Work out the finished part from the listing and answer in its coordinate system (mm). A direction names the side the tool comes from. Give positions to 0.01 mm unless a question says otherwise; leave off trailing zeros. Loops run counter-clockwise (first coordinate to the right, second up) from the corner with the lowest first, then second, coordinate; pieces in that order, holes last.
Autodesk Inventor part; units mm, degrees
ref_plane "YZ Plane" through (0, 0, 0) normal (1, 0, 0) x (0, 1, 0)
ref_plane "XZ Plane" through (0, 0, 0) normal (0, 1, 0) x (-1, 0, 0)
ref_plane "XY Plane" through (0, 0, 0) normal (0, 0, 1) x (1, 0, 0)
sketch "Skizze1" plane through (0, 0, 0) normal (0, 0, 1) x (1, 0, 0)
  line L0 (3.6, 12) -> (48, 12)
  line L1 (48, 12) -> (48, -12)
  line L2 (48, -12) -> (3.6, -12)
  line L3 (-189.6, 0) -> (87.6, 0)
  line L4 (-1, 15) -> (-10, 28.5)
  line L5 (-1, -15) -> (-10, -28.5)
  line L6 (-10, -28.5) -> (-14, -28.5)
  line L7 (-10, 28.5) -> (-14, 28.5)
  arc A0 (-11.6616, 21.5053) -> (-14, 28.5) centre (-33.4005, 18.1259) ccw
  arc A1 (-14, -28.5) -> (-11.6616, -21.5053) centre (-33.4005, -18.1259) ccw
  arc A2 (-11.6616, -21.5053) -> (-11.6616, 21.5053) centre (-150, 0) ccw
  line L8 (-10, 28.5) -> (-10, -28.5) construction
  line L9 (0, 40.0382) -> (0, -40.0382)
  line L10 (-2, 12.5) -> (-2, -9.8115) construction
  arc A3 (0, 12) -> (3.6, 12) centre (1.8, 12) ccw
  arc A4 (3.6, -12) -> (0, -12) centre (1.8, -12) ccw
  line L11 (0, 12) -> (0, 15)
  line L12 (0, 15) -> (-1, 15)
  line L13 (0, -12) -> (0, -15)
  line L14 (0, -15) -> (-1, -15)
  point P0 (0, 0)
  dimension "d2" = 24
  dimension "d51" = 22
  dimension "d52" = 140
  dimension "d54" = 4
  dimension "d55" = 57
  dimension "d59" = 8
  dimension "d60" = 2
  dimension "d64" = 0
  dimension "d73" = 1.8
  dimension "d75" = 48
  dimension "d76" = 30
  dimension "d77" = 1
extrude "Extrusion1" add sketch "Skizze1" along normal blind 12
sketch "Skizze8" plane through (0, 0, 12) normal (0, 0, 1) x (1, 0, 0)
  line L0 (-189.6, 0) -> (87.6, 0)
  arc A0 (-11.6616, -21.5053) -> (-11.6616, 21.5053) centre (-150, 0) ccw
  line L1 (-1, 15) -> (-10, 28.5)
  line L2 (-11.2277, 18.5) -> (-3.3333, 18.5) construction
  point P0 (0, 0)
  point P1 (-5.7805, 18.5)
  point P2 (-5.7805, -18.5)
  point P3 (-7.2805, 18.5)
  dimension "d65" = 18.5
  dimension "d80" = 1.5
hole "Bohrung4" at (-5.7805, 18.5, 12) at (-5.7805, -18.5, 12) direction (0, 0, -1) diameter 1.567 end through all counterbore diameter 5.5 counterbore depth 7
sketch "Skizze2" plane through (0, 0, 0) normal (0, 0, -1) x (-1, 0, 0)
  line L0 (-48, -12) -> (-3.6, -12)
  line L1 (-48, 12) -> (-48, -12)
  line L2 (-48, 12) -> (-3.6, 12)
  line L3 (0, -12) -> (-48, -12)
  line L4 (-48, -12) -> (-48, 12)
  line L5 (-48, 12) -> (0, 12)
  line L6 (-3.6, 12) -> (-48, 12)
  line L7 (0, 12) -> (0, -12)
  point P0 (0, 0)
  point P1 (0, -12.5)
  point P2 (0, 12.5)
  point P3 (-3.6, -12)
extrude "Extrusion2" cut sketch "Skizze2" against normal blind 8
sketch "Skizze3" plane through (0, 0, 8) normal (0, 0, -1) x (-1, 0, 0)
  line L0 (-3.6, -12) -> (-48, -12)
  line L1 (-48, -12) -> (-48, 12)
  line L2 (-48, 12) -> (-3.6, 12)
  line L3 (-48, -12) -> (-44, -12)
  line L4 (-44, -12) -> (-44, 12)
  line L5 (-44, 12) -> (-48, 12)
  line L6 (-48, 12) -> (-48, -12)
  point P0 (0, 0)
  point P1 (0, -12.5)
  point P2 (0, 12.5)
  point P3 (10, -12.5)
  point P4 (-3.6, 12)
  dimension "d9" = 4
extrude "Extrusion3" cut sketch "Skizze3" against normal blind 2
sketch "Skizze4" plane through (0, 0, 12) normal (0, 0, 1) x (1, 0, 0)
  line L0 (48, -12) -> (48, 12)
  line L1 (-26.4, 0) -> (60.4, 0)
  point P0 (0, 0)
  point P1 (46, 0)
  dimension "d12" = 2
hole "Bohrung1" at (46, 0, 12) direction (0, 0, -1) diameter 2 end through all
pattern_linear "Rechteckige Anordnung1" count 5 spacing 5 along (0, 1, 0) of "Bohrung1" first direction both ways yes
sketch "Skizze7" plane through (0, 0, 12) normal (0, 0, 1) x (1, 0, 0)
  line L0 (-1, 15) -> (-3.061, 18.0915)
  line L1 (-10, 28.5) -> (-14, 28.5)
  arc A0 (-11.6616, 21.5053) -> (-14, 28.5) centre (-33.4005, 18.1259) ccw
  arc A1 (-11.6616, -21.5053) -> (-11.6616, 21.5053) centre (-150, 0) ccw
  arc A2 (-14, -28.5) -> (-11.6616, -21.5053) centre (-33.4005, -18.1259) ccw
  line L2 (-14, -28.5) -> (-10, -28.5)
  line L3 (-10, -28.5) -> (-5.1116, -21.1674)
  line L4 (3.6, -12) -> (48, -12)
  line L5 (48, -12) -> (48, 12)
  line L6 (48, 12) -> (3.6, 12)
  line L7 (-3, 28.5) -> (-14, 28.5)
  line L8 (-14, 28.5) -> (-14, -28.5)
  line L9 (-14, -28.5) -> (-3, -28.5)
  line L10 (-3, -28.5) -> (-3, 28.5)
  line L11 (-10, 28.5) -> (-14, 28.5)
  line L12 (-14, -28.5) -> (-10, -28.5)
  line L13 (0, 12) -> (0, 15)
  line L14 (0, 15) -> (-1, 15)
  line L15 (-1, -15) -> (0, -15)
  line L16 (0, -15) -> (0, -12)
  arc A3 (3.6, -12) -> (0, -12) centre (1.8, -12) ccw
  arc A4 (0, 12) -> (3.6, 12) centre (1.8, 12) ccw
  arc A5 (-5.1116, 21.1674) -> (-3.061, 18.0915) centre (-5.7805, 18.5) ccw
  arc A6 (-3.061, -18.0915) -> (-5.1116, -21.1674) centre (-5.7805, -18.5) ccw
  line L17 (-1, -15) -> (0, -15)
  line L18 (0, 15) -> (-1, 15)
  line L19 (-194.4, 0) -> (88.4, 0)
  line L20 (-1, 15) -> (-2, 15)
  line L21 (0, -15) -> (-1, -15)
  line L22 (-2, -15) -> (-1, -15)
  line L23 (-5.1116, 21.1674) -> (-10, 28.5)
  line L24 (-3.061, -18.0915) -> (-1, -15)
  point P0 (0.6841, -13.8749)
  point P1 (0, 0)
  point P2 (-3, -14)
  point P3 (-3, 14)
  dimension "d86" = 3
extrude "Extrusion4" [suppressed]
fillet "Rundung1" radius 2 2 edges at (-1, -15, 6) (-1, 15, 6)
fillet "Rundung2" radius 1 4 edges at (-10, -28.5, 6) (-10, 28.5, 6) (0, -15.0012, 6) (0, 15.0012, 6)
fillet "Rundung3" radius 2.5 4 edges at (-5.1116, -21.1674, 8.5) (-3.061, -18.0915, 8.5) (-5.1116, 21.1674, 8.5) (-3.061, 18.0915, 8.5)
chamfer "Fase1" [suppressed]
sketch "Skizze9" plane through (0, 0, 7) normal (0, 0, 1) x (1, 0, 0)
  arc A0 (-10.4764, 20.7604) -> (-7.2043, 16.343) centre (-8.9101, 18.5) ccw
  line L0 (-12.7002, 28.0952) -> (-9.8914, 24.3034)
  arc A1 (-12.7002, 28.0952) -> (-13.5037, 28.5) centre (-13.5037, 27.5) ccw
  line L1 (-18, 28.5) -> (-13.5037, 28.5)
  arc A2 (-15.6616, 21.5053) -> (-18, 28.5) centre (-37.4005, 18.1259) ccw
  arc A3 (-15.6616, -21.5053) -> (-15.6616, 21.5053) centre (-154, 0) ccw
  arc A4 (-18, -28.5) -> (-15.6616, -21.5053) centre (-37.4005, -18.1259) ccw
  line L2 (-13.5037, -28.5) -> (-18, -28.5)
  arc A5 (-13.5037, -28.5) -> (-12.7002, -28.0952) centre (-13.5037, -27.5) ccw
  line L3 (-9.8914, -24.3034) -> (-12.7002, -28.0952)
  arc A6 (-7.2043, -16.343) -> (-10.4764, -20.7604) centre (-8.9101, -18.5) ccw
  line L4 (-3, 12) -> (-4, 12)
  line L5 (-4, 12) -> (-4, -12)
  line L6 (-4, -12) -> (-3, -12)
  line L7 (-3, -12) -> (-3, 12)
  line L8 (-194.4, 0) -> (88.4, 0)
  line L9 (-3, 15.2723) -> (-3, -15.2723)
  arc A7 (-3, -15.2723) -> (-3.5997, -15.8095) centre (-1.9925, -17) ccw
  arc A8 (-3.5997, 15.8095) -> (-3, 15.2723) centre (-1.9925, 17) ccw
  arc A9 (-3.6446, 15.8702) -> (-7.2043, 16.343) centre (-5.6535, 14.3821) ccw
  arc A10 (-10.4764, 20.7604) -> (-9.8914, 24.3034) centre (-11.9003, 22.8153) ccw
  arc A11 (-9.8914, -24.3034) -> (-10.4764, -20.7604) centre (-11.9003, -22.8153) ccw
  arc A12 (-7.2043, -16.343) -> (-3.6446, -15.8702) centre (-5.6535, -14.3821) ccw
  line L10 (-3.5997, -15.8095) -> (-3.6446, -15.8702)
  line L11 (-3.6446, 15.8702) -> (-3.5997, 15.8095)
  point P0 (0, 0)
  dimension "d88" = 1
  dimension "d89" = 24
extrude "Extrusion5" [suppressed]
sketch "Skizze10" plane through (0, 0, 7) normal (0, 0, 1) x (1, 0, 0)
  arc A0 (-10.4764, 20.7604) -> (-7.2043, 16.343) centre (-8.9101, 18.5) ccw
  arc A1 (-12.7002, 28.0952) -> (-13.5037, 28.5) centre (-13.5037, 27.5) ccw
  line L0 (-18, 28.5) -> (-13.5037, 28.5)
  arc A2 (-15.6616, 21.5053) -> (-18, 28.5) centre (-37.4005, 18.1259) ccw
  arc A3 (-15.6616, -21.5053) -> (-15.6616, 21.5053) centre (-154, 0) ccw
  arc A4 (-18, -28.5) -> (-15.6616, -21.5053) centre (-37.4005, -18.1259) ccw
  line L1 (-13.5037, -28.5) -> (-18, -28.5)
  arc A5 (-13.5037, -28.5) -> (-12.7002, -28.0952) centre (-13.5037, -27.5) ccw
  line L2 (-9.8914, -24.3034) -> (-12.7002, -28.0952)
  arc A6 (-7.2043, -16.343) -> (-10.4764, -20.7604) centre (-8.9101, -18.5) ccw
  line L3 (-4, 12) -> (-5, 12)
  line L4 (-5, 12) -> (-5, -12)
  line L5 (-5, -12) -> (-4, -12)
  line L6 (-4, -12) -> (-4, 12)
  line L7 (-3, 15.2723) -> (-3, -15.2723)
  line L8 (-12.7002, 28.0952) -> (-9.8914, 24.3034)
  arc A7 (-3.5997, 15.8095) -> (-3, 15.2723) centre (-1.9925, 17) ccw
  arc A8 (-3, -15.2723) -> (-3.5997, -15.8095) centre (-1.9925, -17) ccw
  line L9 (-3.6446, 15.8702) -> (-3.5997, 15.8095)
  arc A9 (-3.6446, 15.8702) -> (-7.2043, 16.343) centre (-5.6535, 14.3821) ccw
  arc A10 (-10.4764, 20.7604) -> (-9.8914, 24.3034) centre (-11.9003, 22.8153) ccw
  arc A11 (-9.8914, -24.3034) -> (-10.4764, -20.7604) centre (-11.9003, -22.8153) ccw
  arc A12 (-7.2043, -16.343) -> (-3.6446, -15.8702) centre (-5.6535, -14.3821) ccw
  line L10 (-3.5997, -15.8095) -> (-3.6446, -15.8702)
  point P0 (0, 0)
  dimension "d92" = 1
extrude "Extrusion6" [suppressed]
fillet "Rundung4" [suppressed]
chamfer "Fase3" [suppressed]
properties part number "Kicker Sichel" material "Aluminium 6061"
Item 1: Determine the mould class of faces 1 (the face through (-2.81, 16.39, 8.55)), 2 (the face through (0, 0, 5)), 3 (the face through (-10, 0, 6)), 4 (the face through (26, -12, 10)) for opening direction Y: released by +Y, released by -Y, zero draft, split by the parting line, or undercut.
Item 2: Find section A-A, the plane y = 0. Write down the section's boundary in (x, z).
Item 3: Find section C-C, the plane z = 3. Write down the section's boundary in (x, y).
Item 4: Flat-ended cylindrical pins translate along their axes: pin 1 Ø0.6 at (y, z) = (-3, 8.5) entering from +X; pin 2 Ø2.5 at (x, y) = (46, 5) entering from -Z; pin 3 Ø1.4 at (x, y) = (-5.78, 18.5) entering from +Z; pin 4 Ø12 at (x, y) = (11.5, 3) entering from -Z. Find the tip coordinate at first contact, or state that the pin passes through.
Item 5: Consider line 1 (Y direction, x = 46, z = 11.3); line 2 (Y direction, x = 10.5, z = 11.75); line 3 (X direction, y = 10, z = 11). Determine where each line is inside the solid, lowest interval first.
Item 6: For faces 5 (the face through (-6.6, 22.2, 8.5)), 6 (the face through (17, 0, 12)), 7 (the face through (45, 0, 11)), 8 (the face through (-8.09, -17.01, 8.45)), 9 (the face through (22, 0, 8)), determine the directions among +Z, -Z, +X, -X, +Y, -Y from which every point of the face is accessible in a straight line to the end or side of a thin tool.
Item 7: Find section B-B, the plane x = -2.5. Write down the section's boundary in (y, z), plus the area to 3 significant figures.
Item 8: Find section D-D, the plane y = 18.5. Write down the section's boundary in (x, z), plus the area to 3 significant figures.
Ans:
1. face 1: released by +Y
1. face 2: zero draft
1. face 3: undercut
1. face 4: released by -Y
2. outline: (-10, 0) - (0, 0) - (0, 8) - (44, 8) - (44, 10) - (45, 10) - (45, 12) - (-10, 12) - close; (47, 10) - (48, 10) - (48, 12) - (47, 12) - close
3. outline: (-14, -28.5) - (-10.54, -28.5) arc R1 ccw to (-9.7, -28.05) - (-1.59, -15.89) arc R2 cw to (-0.64, -15.13) arc R1 ccw to (0, -14.2) - (0, 14.2) arc R1 ccw to (-0.64, 15.13) arc R2 cw to (-1.59, 15.89) - (-9.7, 28.05) arc R1 ccw to (-10.54, 28.5) - (-14, 28.5) arc R22 cw to (-11.66, 21.51) arc R140 cw to (-11.66, -21.51) arc R22 cw to start; hole circle Ø1.57 at (-5.78, -18.5); hole circle Ø1.57 at (-5.78, 18.5)
4. pin 1: stops at x = 44
4. pin 2: stops at z = 10
4. pin 3: passes through
4. pin 4: stops at z = 8
5. line 1: y = -12 to -11, -9 to -6, -4 to -1, 1 to 4, 6 to 9, 11 to 12
5. line 2: y = -12 to 12
5. line 3: x = -10.36 to 45, 47 to 48
6. face 5: +Z, +X
6. face 6: +Z, +X, -X, +Y, -Y
6. face 7: +Z, -Z
6. face 8: +Z
6. face 9: -Z, +X, +Y, -Y
7. outline: (-17.25, 0) - (17.25, 0) - (17.25, 5) - (16.32, 5) - (16.32, 12) - (-16.32, 12) - (-16.32, 5) - (-17.25, 5) - close
7. area: 401 mm2
8. outline: (-11.23, 0) - (-6.56, 0) - (-6.56, 5) - (-8.53, 5) - (-8.53, 12) - (-11.23, 12) - close; (-5, 0) - (-3.33, 0) - (-3.33, 5) - (-5, 5) - close
8. area: 50.5 mm2
